The listing builds one solid part. Answer for the finished solid, in the listing's coordinates (mm). Face numbers are marked on the shaded views. Give positions to 0.01 mm unless a question says otherwise; leave off trailing zeros. Order: outer loops, then holes, each group sorted by start corner. A loop starts at its lowest first (then second) coordinate and runs counter-clockwise, first axis right, second up. Notation, with made-up numbers: (-26.5, 61) - (21.5, 61) arc R10 cw to (21.5, 70) - close; hole circle Ø10 at (25.25, -12.5). An arc over 180 degrees is marked (long way). Answer in a Markdown table with one row per item. Add a question column.
```python
from build123d import *

# Parameters (mm, degrees)
SKETCH_W        = 107
SKETCH_H        = 90
PAD_DEPTH       = 30
SKETCH001_W     = 102
SKETCH001_H     = 85
POCKET_DEPTH    = 27
SKETCH002_R     = 3.5
PAD001_DEPTH    = 27
SKETCH003_R     = 3
PAD002_DEPTH    = 5
SKETCH004_R     = 1.5
POCKET001_DEPTH = 5
SKETCH007_R     = 1.5
POCKET003_DEPTH = 10
SKETCH014_W     = 57
SKETCH014_H     = 23
POCKET010_DEPTH = 107.001
SKETCH015_W     = 40
SKETCH015_H     = 23
POCKET011_DEPTH = 2.5


with BuildPart() as part:
    # Sketch → Pad (new body)
    with BuildSketch(Plane.XY):
        with Locations((53.5, 45)):
            Rectangle(SKETCH_W, SKETCH_H)
    extrude(amount=PAD_DEPTH)

    # Sketch001 (on Face6 of Pad) → Pocket (cut)
    with BuildSketch(Plane.XY.offset(30)):
        with Locations((53.5, 45)):
            Rectangle(SKETCH001_W, SKETCH001_H)
    extrude(amount=-POCKET_DEPTH, mode=Mode.SUBTRACT)

    # Sketch002 (on Face11 of Pocket) → Pad001 (join)
    with BuildSketch(Plane.XY.offset(3)):
        with Locations((3.5, 86.5)):
            Circle(SKETCH002_R)
        with Locations((3.5, 3.5)):
            Circle(SKETCH002_R)
        with Locations((103.5, 86.5)):
            Circle(SKETCH002_R)
        with Locations((103.5, 3.5)):
            Circle(SKETCH002_R)
    extrude(amount=PAD001_DEPTH)

    # Sketch003 (on Face23 of Pad001) → Pad002 (join)
    with BuildSketch(Plane.XY.offset(3)):
        with Locations((6.891, 77.04)):
            Circle(SKETCH003_R)
        with Locations((6.891, 12.96)):
            Circle(SKETCH003_R)
        with Locations((100.109, 77.04)):
            Circle(SKETCH003_R)
        with Locations((100.109, 12.96)):
            Circle(SKETCH003_R)
    extrude(amount=PAD002_DEPTH)

    # Sketch004 (on Face39 of Pad002) → Pocket001 (cut)
    with BuildSketch(Plane.XY.offset(8)):
        with Locations((6.891, 77.04)):
            Circle(SKETCH004_R)
        with Locations((100.109, 77.04)):
            Circle(SKETCH004_R)
        with Locations((100.109, 12.96)):
            Circle(SKETCH004_R)
        with Locations((6.891, 12.96)):
            Circle(SKETCH004_R)
    extrude(amount=-POCKET001_DEPTH, mode=Mode.SUBTRACT)

    # Sketch007 (on Face17 of Pad001) → Pocket003 (cut)
    with BuildSketch(Plane.XY.offset(30)):
        with Locations((3.5, 86.5)):
            Circle(SKETCH007_R)
        with Locations((103.5, 86.5)):
            Circle(SKETCH007_R)
        with Locations((103.5, 3.5)):
            Circle(SKETCH007_R)
        with Locations((3.5, 3.5)):
            Circle(SKETCH007_R)
    extrude(amount=-POCKET003_DEPTH, mode=Mode.SUBTRACT)

    # Sketch014 → Pocket010 (cut, through all)
    with BuildSketch(Plane(origin=(0, 0, 0), x_dir=(0, -1, 0), z_dir=(-1, 0, 0))):
        with Locations((-45, 18.5)):
            Rectangle(SKETCH014_W, SKETCH014_H)
    extrude(amount=-POCKET010_DEPTH, mode=Mode.SUBTRACT)

    # Sketch015 (on Face1 of Pocket010) → Pocket011 (cut)
    with BuildSketch(Plane.XZ):
        with Locations((57.5, 18.5)):
            Rectangle(SKETCH015_W, SKETCH015_H)
    extrude(amount=-POCKET011_DEPTH, mode=Mode.SUBTRACT)


solid = part.part
```
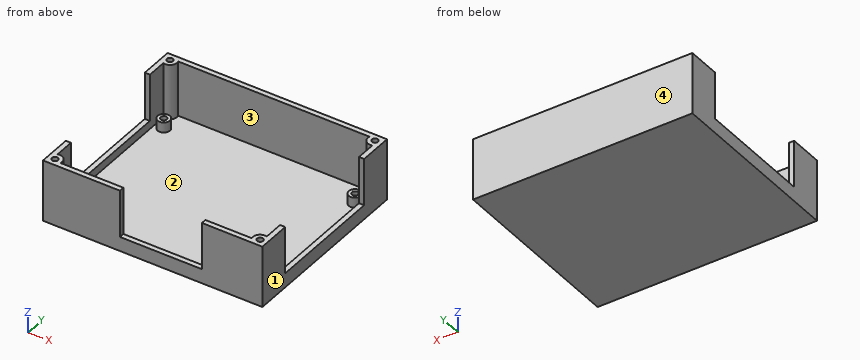
(1) Straight lines are drawn through the part: line 1 (X direction, y = 86.5, z = 23.75); line 2 (Y direction, x = 103.5, z = 23.5); line 3 (Y direction, x = 86.5, z = 12.25). For each, find the intervals that lie inside material, in ascending order.
(2) Find section D-D, the plane x = 53.5. Write down the section's boundary in (y, z), plus the area to 4 significant figures.
(3) Each of these flat-tipped pins is pushed along its axis until it touches: P1, Ø5, axis at x = 82, y = 35, coming from the +Z side; P2, Ø6.5, axis at x = 100, y = 78, coming from the +Z side; P3, Ø2, axis at x = 1.5, y = 55, coming from the +Z side. Where does it stop, or does it pass through?
(4) Find section C-C, the plane y = 77.04. Write down the section's boundary in (x, z).
(5) The mould has two halves that part along Y. Classify the marked faces 1, 2, 3 and 4: +Y half, -Y half, draft (parallel to the pull), parting line (faces both ways), or undercut.
(6) Find section A-A, the plane z = 24.5. Write down the section's boundary in (x, y), plus the area to 3 significant figures.
(7) Find section B-B, the plane x = 90.5. Write down the section's boundary in (y, z), plus the area to 3 significant figures.
Answer key:
| question | item | result |
|---|---|---|
| 1 | line 1 | 0 to 2, 5 to 7, 100 to 102, 105 to 107 |
| 1 | line 2 | 0 to 2, 5 to 7, 83 to 85, 88 to 90 |
| 1 | line 3 | 0 to 2.5, 87.5 to 90 |
| 2 | outline | (0, 0) - (90, 0) - (90, 30) - (87.5, 30) - (87.5, 3) - (2.5, 3) - (2.5, 7) - (0, 7) - close |
| 2 | area | 347.5 mm² |
| 3 | P1 | z = 3 |
| 3 | P2 | z = 8 |
| 3 | P3 | z = 7 |
| 4 | outline | (0, 0) - (107, 0) - (107, 30) - (104.5, 30) - (104.5, 3) - (103.11, 3) - (103.11, 8) - (101.61, 8) - (101.61, 3) - (98.61, 3) - (98.61, 8) - (97.11, 8) - (97.11, 3) - (9.89, 3) - (9.89, 8) - (8.39, 8) - (8.39, 3) - (5.39, 3) - (5.39, 8) - (3.89, 8) - (3.89, 3) - (2.5, 3) - (2.5, 30) - (0, 30) - close |
| 5 | face 1 | draft |
| 5 | face 2 | undercut |
| 5 | face 3 | undercut |
| 5 | face 4 | +Y half |
| 6 | outline | (0, 0) - (37.5, 0) - (37.5, 2.5) - (6.85, 2.5) arc R3.5 ccw to (2.5, 6.85) - (2.5, 16.5) - (0, 16.5) - close; (0, 73.5) - (2.5, 73.5) - (2.5, 83.15) arc R3.5 ccw to (6.85, 87.5) - (100.15, 87.5) arc R3.5 ccw to (104.5, 83.15) - (104.5, 73.5) - (107, 73.5) - (107, 90) - (0, 90) - close; (77.5, 0) - (107, 0) - (107, 16.5) - (104.5, 16.5) - (104.5, 6.85) arc R3.5 ccw to (100.15, 2.5) - (77.5, 2.5) - close; hole circle Ø3 at (3.5, 3.5); hole circle Ø3 at (3.5, 86.5); hole circle Ø3 at (103.5, 3.5); hole circle Ø3 at (103.5, 86.5) |
| 6 | area | 617 mm² |
| 7 | outline | (0, 0) - (90, 0) - (90, 30) - (87.5, 30) - (87.5, 3) - (2.5, 3) - (2.5, 30) - (0, 30) - close |
| 7 | area | 405 mm² |
